Work out the finished part from the listing and answer in its coordinate system (mm). Give positions to 0.01 mm unless a question says otherwise; leave off trailing zeros. Order: outer loops, then holes, each group sorted by start corner. A loop starts at its lowest first (then second) coordinate and runs counter-clockwise, first axis right, second up. Notation, with made-up numbers: M 75,32 L 81,32 A21 cw 81,41 Z; hole C 65,-39.5 d2. An arc over 180 degrees is marked long. One line per item, written item: value.
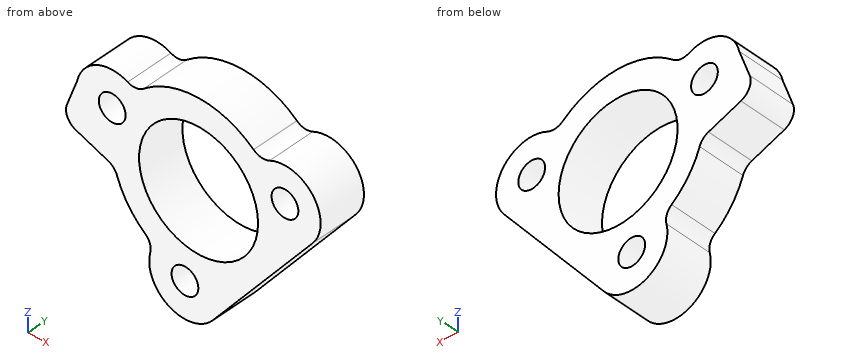
from build123d import *

# Parameters (mm, degrees)
F0_R     = 20
F1_DEPTH = 16
F2_D     = 9


with BuildPart() as f1:
    # F0 (on Front) → F1 (new body)
    with BuildSketch(Plane.XZ):
        with BuildLine():
            ThreePointArc((-30.3928510428, -6.3968226045), (-28.562967972, -7.5906259687), (-27.4168456036, -9.4507447933))
            ThreePointArc((-27.4168456036, -9.4507447933), (-23.6605152057, -16.7684233069), (-18.0006967285, -22.7370824269))
            ThreePointArc((-18.0006967285, -22.7370824269), (-16.3768862519, -25.0288069118), (-16.2448023697, -27.8343933793))
            ThreePointArc((-16.2448023697, -27.8343933793), (-9.9005108102, -41.4165554271), (4.7436597925, -38.2113364568))
            Line((4.7436597925, -38.2113364568), (38.3625894042, 3.3045841264))
            ThreePointArc((38.3625894042, 3.3045841264), (38.4530723792, 18.2951469617), (23.8486607741, 21.6769102527))
            ThreePointArc((23.8486607741, 21.6769102527), (21.076921319, 21.222793559), (18.4976673308, 22.3346435682))
            ThreePointArc((18.4976673308, 22.3346435682), (0, 29), (-18.4976673308, 22.3346435682))
            ThreePointArc((-18.4976673308, 22.3346435682), (-21.076921319, 21.222793559), (-23.8486607741, 21.6769102527))
            ThreePointArc((-23.8486607741, 21.6769102527), (-34.2706182279, 21.6549260816), (-40.7447903835, 13.4877493741))
            Line((-40.7447903835, 13.4877493741), (-44.2468641961, 4.1210274816))
            ThreePointArc((-44.2468641961, 4.1210274816), (-44.1133096043, 0.296524362), (-41.3145401562, -2.3133703709))
            Line((-41.3145401562, -2.3133703709), (-30.3928510428, -6.3968226045))
        make_face()
        Circle(F0_R, mode=Mode.SUBTRACT)
    extrude(amount=F1_DEPTH)

    # F2 (through all)
    with Locations(Plane(origin=(0, 0, 0), x_dir=(1, 0, 0), z_dir=(0, 1, 0))):
        with Locations((29.0368378667, -10.856428819), (-29.0368378667, -10.856428819), (-4.582091745, 30.6594917642)):
            Hole(F2_D / 2)


solid = f1.part
(1) Section B-B, the plane z = 0 is taken. Give the vertices of the cut face in (x, y), then the cut area to 3 significant figures.
Findings:
outline: M -43.97,-16 L -20,-16 L -20,0 L -43.97,0 Z; M 20,-16 L 35.69,-16 L 35.69,0 L 20,0 Z
area: 634 mm^2
(2) Find the intervals of material crossed by probe 1 along X at (y, z) = (-14.25, 12.5); probe 2 along X at (y, z) = (-8.5, 7) (3 decimals); probe 3 along Z at (x, y) = (-5.5, -0.5), in increasing order. Write a range as from..to.
Findings:
probe 1: x = -41.11..-33.23, -24.85..-15.61, 15.61..24.85, 33.23..40.92
probe 2: x = -43.17..-31.356, -26.718..-18.735, 18.735..26.718, 31.356..40.4
probe 3: z = -42.62..-35.06, -26.25..-19.23, 19.23..28.47
(3) Section D-D, the plane x = -35.5 is taken. Give the vertices of the cut face in (y, z), then the cut area to 3 significant figures.
Findings:
outline: M -16,-4.49 L 0,-4.49 L 0,20.97 L -16,20.97 Z
area: 407 mm^2
(4) Given P1, Ø1, axis at x = 1.5, y = -10.5, coming from the +Z side; P2, Ø8, axis at y = -4.5, z = 2.5, coming from the +X side; P3, Ø5.5, axis at x = -4.58, z = -30.66, coming from the +Y side; P4, Ø1, axis at x = -27.5, y = -7, coming from the +Z side, each flat-ended and moving along its own axis, determine where each tip first touches the part or whether it passes through.
Findings:
P1: stops at z = 28.98
P2: stops at x = 40.22
P3: passes through
P4: stops at z = 22.81
(5) Section C-C, the plane y = -14.75 is taken. Give the vertices of the cut face in (x, z).
Findings:
outline: M -44.25,4.12 A5 ccw -41.31,-2.31 L -30.39,-6.4 A5 cw -27.42,-9.45 A29 ccw -18,-22.74 A5 cw -16.24,-27.83 A12 ccw 4.74,-38.21 L 38.36,3.3 A12 ccw 23.85,21.68 A5 cw 18.5,22.33 A29 ccw -18.5,22.33 A5 cw -23.85,21.68 A12 ccw -40.74,13.49 Z; hole C -29.04,10.86 d9; hole C 0,0 d40; hole C -4.58,-30.66 d9; hole C 29.04,10.86 d9
(6) Section A-A, the plane x = 16.5 is taken. Give the vertices of the cut face in (y, z).
Findings:
outline: M -16,-23.69 L 0,-23.69 L 0,-11.3 L -16,-11.3 Z; M -16,11.3 L 0,11.3 L 0,23.85 L -16,23.85 Z
